Input: part model. Units: mm. Frame: model coordinates. Face numbers are marked on the shaded views. A direction names the side the tool comes from. Coordinates: 2 decimals unless noted, no trailing zeros. Write each loop counter-clockwise with the first axis right and the second up, starting at its lowest first coordinate (ties: lowest second). Pieces come first, ordered by that corner, then holes. Notation, with made-up numbers: (4.5, 42.25) - (47.5, 42.25) arc R12 cw to (47.5, 57.25) - close; hole circle Ø9 at (54, 54.25). An arc over 180 degrees is marked (long way). Use CSV: the item, a comma, the result in double quotes.
```python
from build123d import *

# Parameters (mm, degrees)
F0_W       = 80
F0_H       = 100
F0_R       = 5
F0_R_2     = 20
F1_DEPTH   = 5
F2_DEPTH   = 12
F4_DEPTH   = 3
F5_W       = 3
F5_H       = 60
F6_DEPTH   = 70
F7_SIZE2   = 40
F7_SIZE    = 65
F8_SIZE2   = 6.5
F8_SIZE    = 4
F8_2_SIZE2 = 6.5
F8_2_SIZE  = 4
F9_R       = 5
F10_DEPTH  = 60


with BuildPart() as f1:
    # F0 (on Top) → F1 (new body)
    with BuildSketch(Plane.XY):
        Rectangle(F0_W, F0_H)
        with Locations((-27.5, -40)):
            Circle(F0_R, mode=Mode.SUBTRACT)
        with Locations((27.5, -40)):
            Circle(F0_R, mode=Mode.SUBTRACT)
        with Locations((-27.5, 40)):
            Circle(F0_R, mode=Mode.SUBTRACT)
        Circle(F0_R_2, mode=Mode.SUBTRACT)
        with Locations((27.5, 40)):
            Circle(F0_R, mode=Mode.SUBTRACT)
        Circle(F0_R_2)
    extrude(amount=F1_DEPTH)

    # F0 (on Top) → F2 (join)
    with BuildSketch(Plane.XY):
        Circle(F0_R_2)
    extrude(amount=F2_DEPTH)

    # F3 (on face) → F4 (join)
    with BuildSketch(Plane.XY.offset(12)):
        with BuildLine():
            Line((-18, -30), (18, -30))
            Line((18, -30), (18, -8.7177978871))
            ThreePointArc((18, -8.7177978871), (0, -20), (-18, -8.7177978871))
            Line((-18, -8.7177978871), (-18, -30))
        make_face()
        with BuildLine():
            ThreePointArc((-18, -8.7177978871), (0, -20), (18, -8.7177978871))
            Line((18, -8.7177978871), (18, 8.7177978871))
            ThreePointArc((18, 8.7177978871), (0, 20), (-18, 8.7177978871))
            Line((-18, 8.7177978871), (-18, -8.7177978871))
        make_face()
        with BuildLine():
            ThreePointArc((-18, 8.7177978871), (0, 20), (18, 8.7177978871))
            Line((18, 8.7177978871), (18, 30))
            Line((18, 30), (-18, 30))
            Line((-18, 30), (-18, 8.7177978871))
        make_face()
    extrude(amount=F4_DEPTH)

    # F5 (on face) → F6 (join)
    with BuildSketch(Plane.XY.offset(15)):
        with Locations((-16.5, 0)):
            Rectangle(F5_W, F5_H)
        with Locations((16.5, 0)):
            Rectangle(F5_W, F5_H)
    extrude(amount=F6_DEPTH)

    # F7
    f7_edges = [f1.edges().sort_by_distance(p)[0] for p in [
        (16.5, -30, 85),
        (-16.5, -30, 85),
    ]]
    f7_side = f1.faces().sort_by_distance((-17.186059, -30, 48.5))[0]
    chamfer(f7_edges, length=F7_SIZE, length2=F7_SIZE2, reference=f7_side)

    # F8
    f8_edges = [f1.edges().sort_by_distance(p)[0] for p in [
        (16.5, 30, 85),
    ]]
    f8_side = f1.faces().sort_by_distance((16.5, 20, 85))[0]
    chamfer(f8_edges, length=F8_SIZE, length2=F8_SIZE2, reference=f8_side)

    # F8#2
    f8_2_edges = [f1.edges().sort_by_distance(p)[0] for p in [
        (-16.5, 30, 85),
    ]]
    f8_2_side = f1.faces().sort_by_distance((-16.5, 20, 85))[0]
    chamfer(f8_2_edges, length=F8_2_SIZE, length2=F8_2_SIZE2, reference=f8_2_side)

    # F9 (on face) → F10 (cut)
    with BuildSketch(Plane(origin=(-18, 0, 0), x_dir=(0, -1, 0), z_dir=(-1, 0, 0))):
        with Locations((-18, 77)):
            Circle(F9_R)
    extrude(amount=-F10_DEPTH, mode=Mode.SUBTRACT)


solid = f1.part
```
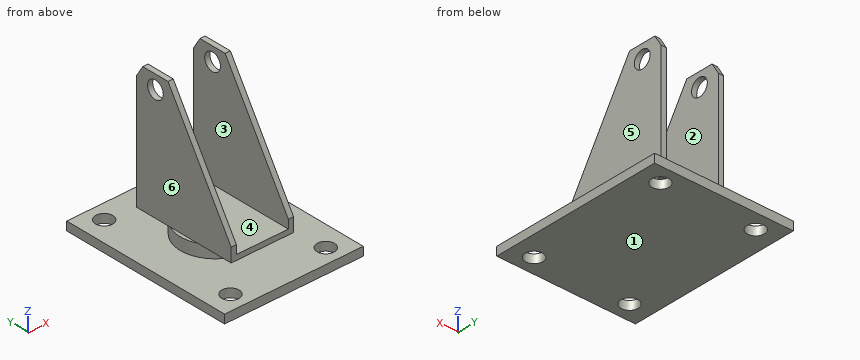
(1) Ray query, probe 1 along Z at (x, y) = (-15.8, 18); probe 2 along Y at (x, z) = (-27, 2); probe 3 along X at (y, z) = (-4, 32). Return the intervals inside material, ascending. Write a range as from..to.
Check values:
probe 1,"0..5, 12..72, 82..85"
probe 2,"-50..-44.97, -35.03..35.03, 44.97..50"
probe 3,"-18..-15, 15..18"
(2) Draft query along X for the marked faces 3, 4, 5 and 6. Return one class per face: pulls with the +X half, pulls with the -X half, needs draft (parallel to the pull), parting line crosses it, or undercut.
Check values:
face 3,"undercut"
face 4,"undercut"
face 5,"pulls with the +X half"
face 6,"pulls with the -X half"
(3) Cut plane D-D on x = 0. Return loops of the section in (y, z), and give its area (3 significant figures).
Check values:
outline,"(-50, 0) - (50, 0) - (50, 5) - (20, 5) - (20, 12) - (30, 12) - (30, 15) - (-30, 15) - (-30, 12) - (-20, 12) - (-20, 5) - (-50, 5) - close"
area,"960 mm^2"
(4) Reachability of the marked faces 1 and 2 from +Z, -Z, +X, -X, +Y, -Y: full face, straight path, thin tool, end or side. Return the list, or none.
Check values:
face 1,"-Z, +X, -X, +Y, -Y"
face 2,"+Z, +Y, -Y"
(5) Cut plane C-C on y = -40. Return loops of the section in (x, z).
Check values:
outline,"(-40, 0) - (-32.5, 0) - (-32.5, 5) - (-40, 5) - close; (-22.5, 0) - (22.5, 0) - (22.5, 5) - (-22.5, 5) - close; (32.5, 0) - (40, 0) - (40, 5) - (32.5, 5) - close"
(6) Cut plane B-B on z = 59. Return loops of the section in (x, y).
Check values:
outline,"(-18, -6) - (-15, -6) - (-15, 30) - (-18, 30) - close; (15, -6) - (18, -6) - (18, 30) - (15, 30) - close"
(7) Pin query (flat end, axial travel): pin 1 Ø8 at (y, z) = (7.5, 35) entering from -X; pin 2 Ø6.5 at (x, z) = (-4.5, 17) entering from -Y; pin 3 Ø16 at (x, y) = (-27.5, 40) entering from +Z. Return the tip coordinate at first contact, or that it passes through.
Check values:
pin 1,"x = -18"
pin 2,"y = -30"
pin 3,"z = 5"
(8) Cut plane A-A on x = -27.5. Return loops of the section in (y, z), and give its area (3 significant figures).
Check values:
outline,"(-50, 0) - (-45, 0) - (-45, 5) - (-50, 5) - close; (-35, 0) - (35, 0) - (35, 5) - (-35, 5) - close; (45, 0) - (50, 0) - (50, 5) - (45, 5) - close"
area,"400 mm^2"
